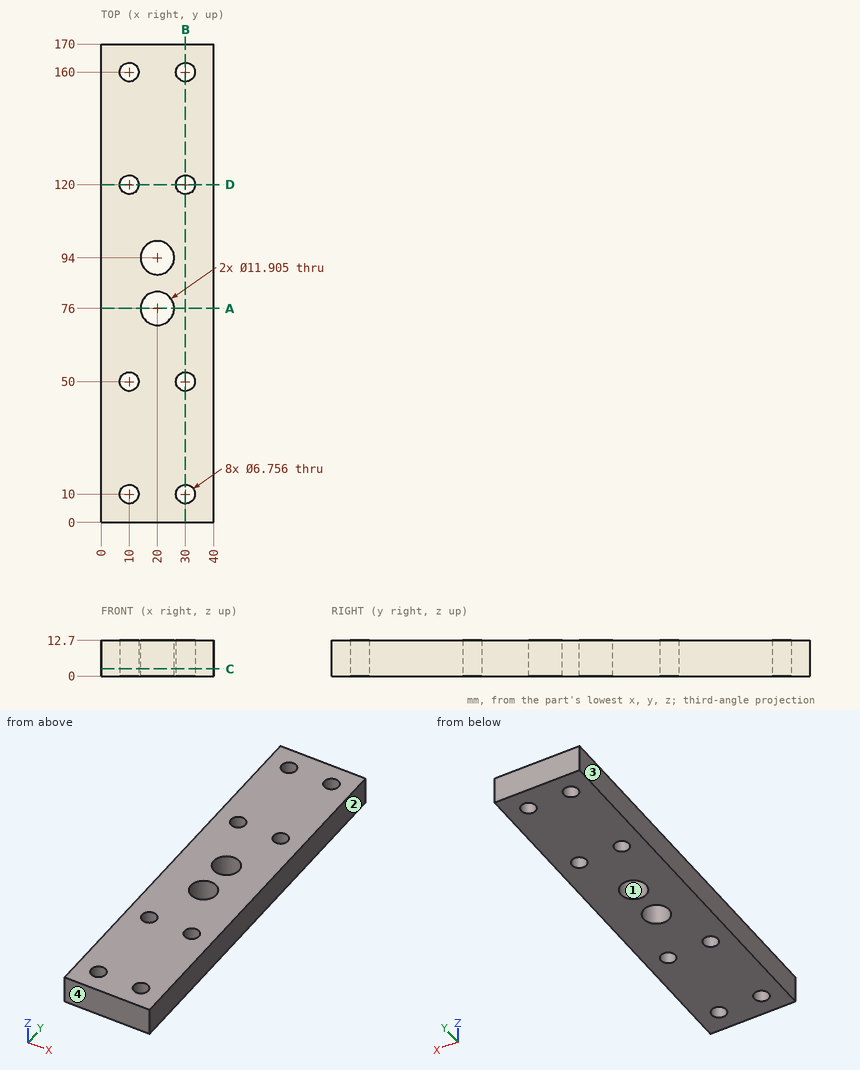
Can you work these out from the drawing? Everything is in mm from the part's minimum corner. Give positions to 0.01 mm unless a question says otherwise; leave off trailing zeros. Loops run counter-clockwise (first coordinate to the right, second up) from the corner with the lowest first, then second, coordinate; pieces in that order, holes last. Notation, with made-up numbers: M 56,57 L 76,57 A17 ccw 76,90 Z; hole C -39,72.25 d10. An arc over 180 degrees is marked long. Put each result on its own line as item: value. Start each with the question number.
(1) I want a section at B-B on x = 30. Please give me the cut outline in (y, z), then the cut area to 3 significant figures.
(2) Will this pin go through, and if not, where does the flat tip stop? pin 1 Ø7 at (x, y) = (20, 76) entering from +Z.
(3) I want a section at A-A on y = 76. Please give me the cut outline in (x, z), then the cut area to 3 significant figures.
(4) I want a section at C-C on z = 2.5. State how many separate pieces and enclosed holes the cut face has, then the cut area to 3 significant figures.
(5) I want a section at D-D on y = 120. Please give me the cut outline in (x, z).
(6) I need wall thicknesses on line 1 along Y through (x, z) = (20, 7); line 2 along X through (y, z) = (8, 6.75); line 3 along Y through (x, z) = (21, 4.75). Which ranges of each line are inside material? Lowest first, please. Write a range as [from, to].
(7) If we mould it in two halves opening along X, with no side actions, what happens to the marked faces 1, 2, 3 and 4? For each: +X half, -X half, draft (parallel to the pull), parting line (faces both ways), or undercut.
Answer block:
1. outline: M 0,0 L 6.62,0 L 6.62,12.7 L 0,12.7 Z; M 13.38,0 L 46.62,0 L 46.62,12.7 L 13.38,12.7 Z; M 53.38,0 L 116.62,0 L 116.62,12.7 L 53.38,12.7 Z; M 123.38,0 L 156.62,0 L 156.62,12.7 L 123.38,12.7 Z; M 163.38,0 L 170,0 L 170,12.7 L 163.38,12.7 Z
1. area: 1,820 mm^2
2. pin 1: through
3. outline: M 0,0 L 14.05,0 L 14.05,12.7 L 0,12.7 Z; M 25.95,0 L 40,0 L 40,12.7 L 25.95,12.7 Z
3. area: 357 mm^2
4. separate pieces: 1
4. enclosed holes: 10
4. area: 6,290 mm^2
5. outline: M 0,0 L 6.62,0 L 6.62,12.7 L 0,12.7 Z; M 13.38,0 L 26.62,0 L 26.62,12.7 L 13.38,12.7 Z; M 33.38,0 L 40,0 L 40,12.7 L 33.38,12.7 Z
6. line 1: [0, 70.05], [81.95, 88.05], [99.95, 170]
6. line 2: [0, 7.28], [12.72, 27.28], [32.72, 40]
6. line 3: [0, 70.13], [81.87, 88.13], [99.87, 170]
7. face 1: undercut
7. face 2: +X half
7. face 3: -X half
7. face 4: draft
